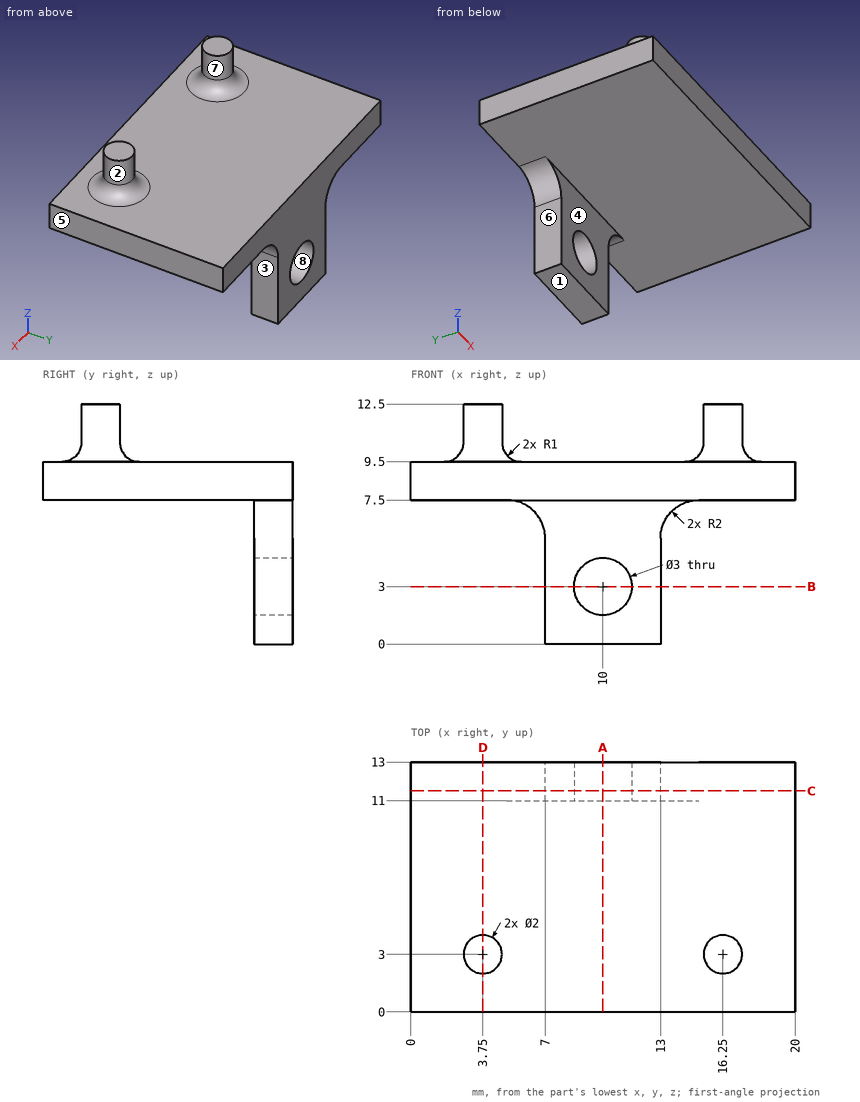
Check sheet for the drawn part. Datum: minimum x, y, z corner. Units: mm. A direction names the side the tool comes from. Round coordinates to 2 decimals unless told otherwise and drop trailing zeros. Order: outer loops, then holes, each group sorted by start corner. A loop starts at its lowest first (then second) coordinate and runs counter-clockwise, first axis right, second up. Notation, with made-up numbers: (3.25, 30) -> (54.25, 30) arc R23 ccw to (54.25, 67) -> close; hole circle Ø3 at (-37.75, -24). An arc over 180 degrees is marked (long way). Put each result on its own line as item: value. Start each with the question number.
(1) Section check C-C (y = 11.5). Enter the section's corners in (x, z).
(2) Section check A-A (x = 10). Enter the section's corners in (y, z).
(3) Section check B-B (z = 3). Enter the section's corners in (x, y), then the cut area to 3 significant figures.
(4) Depth check by flat-ended pin: pin 1 Ø1.6 at (y, z) = (12, 2.5) entering from -X; pin 2 Ø1.5 at (x, y) = (16, 6.5) entering from +Z; pin 3 Ø1.8 at (x, z) = (10, 3) entering from +Y; pin 4 Ø1 at (y, z) = (11.5, 3) entering from +X. Enter the tip coordinate at first touch or a pass-through.
(5) Tool access check on the marked faces 1, 2, 3 and 4. Record the directions out of +Z, -Z, +X, -X, +Y, -Y that give a thin tool (end or side, any length) a straight path to the whole face; none if there is none.
(6) Material ranges on line 1 along X through (y, z) = (12, 3); line 2 along Z through (x, y) = (17.5, 8); line 3 along Y through (x, z) = (10.75, 4.5), recorded low to high.
(7) Draft check along X on the marked faces 5, 6, 7 and 8. Enter one of: +X half, -X half, draft (parallel to the pull), parting line (faces both ways), or undercut.
(8) Section check D-D (x = 3.75). Enter the section's corners in (y, z), then the cut area to 3 significant figures.
Completed:
1. outline: (0, 7.5) -> (5, 7.5) arc R2 cw to (7, 5.5) -> (7, 0) -> (13, 0) -> (13, 5.5) arc R2 cw to (15, 7.5) -> (20, 7.5) -> (20, 9.5) -> (0, 9.5) -> close; hole circle Ø3 at (10, 3)
2. outline: (0, 7.5) -> (11, 7.5) -> (11, 4.5) -> (13, 4.5) -> (13, 9.5) -> (0, 9.5) -> close; (11, 0) -> (13, 0) -> (13, 1.5) -> (11, 1.5) -> close
3. outline: (7, 11) -> (8.5, 11) -> (8.5, 13) -> (7, 13) -> close; (11.5, 11) -> (13, 11) -> (13, 13) -> (11.5, 13) -> close
3. area: 6.00 mm2
4. pin 1: stops at x = 7
4. pin 2: stops at z = 9.5
4. pin 3: passes through
4. pin 4: stops at x = 13
5. face 1: -Z, +X, -X, +Y, -Y
5. face 2: +Z
5. face 3: -Z, +X, +Y, -Y
5. face 4: -Z, +X, -X, -Y
6. line 1: x = 7 to 8.5, 11.5 to 13
6. line 2: z = 7.5 to 9.5
6. line 3: y = 11 to 13
7. face 5: +X half
7. face 6: -X half
7. face 7: undercut
7. face 8: undercut
8. outline: (0, 7.5) -> (13, 7.5) -> (13, 9.5) -> (5, 9.5) arc R1 cw to (4, 10.5) -> (4, 12.5) -> (2, 12.5) -> (2, 10.5) arc R1 cw to (1, 9.5) -> (0, 9.5) -> close
8. area: 32.4 mm2
